from build123d import *

# Parameters (mm, degrees)
ESBO_O2_W                = 15
ESBO_O2_H                = 15
RESSALTO_EXTRUS_O2_DEPTH = 5
ESBO_O3_W                = 10
ESBO_O3_H                = 10
RESSALTO_EXTRUS_O3_DEPTH = 35
FILETE1_R                = 4
ESBO_O4_W                = 6
ESBO_O4_H                = 6
CORTE_EXTRUS_O1_DEPTH    = 46.276925691


with BuildPart() as part:
    # Esboço2 → Ressalto-extrusão2 (new body)
    with BuildSketch(Plane(origin=(0, 0, 0), x_dir=(1, 0, 0), z_dir=(0, 1, 0))):
        with Locations((7.5, -7.5)):
            Rectangle(ESBO_O2_W, ESBO_O2_H)
    extrude(amount=RESSALTO_EXTRUS_O2_DEPTH)

    # Esboço3 → Ressalto-extrusão3 (add)
    with BuildSketch(Plane(origin=(0, 5, 0), x_dir=(1, 0, 0), z_dir=(0, 1, 0))):
        with Locations((7.5, -7.5)):
            Rectangle(ESBO_O3_W, ESBO_O3_H)
    extrude(amount=RESSALTO_EXTRUS_O3_DEPTH)

    # Filete1
    filete1_edges = [part.edges().sort_by_distance(p)[0] for p in [
        (0, 2.5, 0),
        (15, 2.5, 0),
        (15, 2.5, 15),
        (0, 2.5, 15),
    ]]
    fillet(filete1_edges, radius=FILETE1_R)

    # Esboço4 → Corte-extrusão1 (cut, through all)
    with BuildSketch(Plane(origin=(0, 40, 0), x_dir=(1, 0, 0), z_dir=(0, 1, 0))):
        with Locations((7.5, -7.5)):
            Rectangle(ESBO_O4_W, ESBO_O4_H)
    extrude(amount=-CORTE_EXTRUS_O1_DEPTH, mode=Mode.SUBTRACT)


solid = part.part
Verification items for the finished model (mm, model axes). A direction names the side the tool comes from. Coordinates: 2 decimals unless noted, no trailing zeros. Order: outer loops, then holes, each group sorted by start corner. A loop starts at its lowest first (then second) coordinate and runs counter-clockwise, first axis right, second up. Notation, with made-up numbers: (4, -12.75) -> (46, -12.75) arc R29 cw to (46, 11.25) -> close; hole circle Ø7 at (59.5, 28.25). An arc over 180 degrees is marked (long way). Put each result on its own line as item: value. Start each with the question number.
1. Cross-section at D-D, the plane x = 3. Record the boundary of the cut face in (y, z), then the cut area to 3 significant figures.
2. Cross-section at A-A, the plane y = 14. Record the boundary of the cut face in (x, z).
3. Access from +Z, -Z, +X, -X, +Y, -Y to the whole of each face (thin tool, end or side, straight path). Record for faces 4 (the flat face through (7, 20, 4.5)), 5 (the flat face through (2.5, 22, 8)), 6 (the flat face through (12.5, 22, 8)).
4. Go/stop test with flat-tipped pins: pin 1 Ø5 at (y, z) = (23.5, 7) entering from -X; pin 2 Ø5 at (x, y) = (12, 36) entering from -Z; pin 3 Ø5 at (y, z) = (17.5, 8.5) entering from +X; pin 4 Ø1 at (x, z) = (8.5, 8.5) entering from +Y. Record where each tip stops, or that it passes through.
5. Material ranges on L1, parallel to Z at x = 9.75, y = 23; L2, parallel to X at y = 3, z = 7.75, recorded low to high. Write a range as [from, to].
6. Cross-section at C-C, the plane z = 11.5. Record the boundary of the cut face in (x, y).
7. Mould release check, pull along Z, two halves, no side actions. Record for faces 1 (the flat face through (7, 5, 2)), 2 (the flat face through (10.5, 20, 8)), 3 (the flat face through (7, 22, 2.5)): released by +Z, released by -Z, zero draft, split by the parting line, or undercut.
8. Cross-section at B-B, the plane x = 9. Record the boundary of the cut face in (y, z), then the cut area to 3 significant figures.
Computed:
1. outline: (0, 0.13) -> (5, 0.13) -> (5, 2.5) -> (40, 2.5) -> (40, 12.5) -> (5, 12.5) -> (5, 14.87) -> (0, 14.87) -> close
1. area: 424 mm2
2. outline: (2.5, 2.5) -> (12.5, 2.5) -> (12.5, 12.5) -> (2.5, 12.5) -> close; hole (4.5, 4.5) -> (10.5, 4.5) -> (10.5, 10.5) -> (4.5, 10.5) -> close
3. face 4: +Y, -Y
3. face 5: +Z, -Z, -X, +Y
3. face 6: +Z, -Z, +X, +Y
4. pin 1: x = 2.5
4. pin 2: z = 2.5
4. pin 3: x = 12.5
4. pin 4: through
5. L1: [2.5, 4.5], [10.5, 12.5]
5. L2: [0, 4.5], [10.5, 15]
6. outline: (0.03, 0) -> (14.97, 0) -> (14.97, 5) -> (12.5, 5) -> (12.5, 40) -> (2.5, 40) -> (2.5, 5) -> (0.03, 5) -> close
7. face 1: zero draft
7. face 2: undercut
7. face 3: released by -Z
8. outline: (0, 0) -> (5, 0) -> (5, 2.5) -> (40, 2.5) -> (40, 4.5) -> (0, 4.5) -> close; (0, 10.5) -> (40, 10.5) -> (40, 12.5) -> (5, 12.5) -> (5, 15) -> (0, 15) -> close
8. area: 185 mm2
